Can you work these out from the model? Positions are in its coordinate system, mm. Round coordinates to 2 decimals unless told otherwise and drop trailing zeros. Order: outer loops, then holes, each group sorted by start corner. A loop starts at its lowest first (then second) coordinate and runs counter-clockwise, first axis right, second up.
Q1. If we section it at C-C (y = 7.5): Please give me the cut outline in (x, z), plus the area to 3 significant figures.
Q2. If we section it at A-A (z = 0): Please give me the cut outline in (x, y).
Q3. If we section it at B-B (y = 3.25): Please give me the cut outline in (x, z), plus the area to 3 significant figures.
Q4. If I drill on line 1 (X direction, y = 7.5, z = 0); line 2 (Z direction, x = 1, y = 1.25); line 3 (Z direction, x = 1.5, y = 8), over which ranges is the centre line in solid material (lowest first)?
from build123d import *
from build123d.topology import SkipClean

# Parameters (mm, degrees)
SKETCH1_R                   = 4
BOSS_EXTRUDE1_DEPTH         = 7
F_3_8_24_TAPPED_HOLE6_D     = 8.4328
F_3_8_24_TAPPED_HOLE6_DEPTH = 15.3
F_3_8_24_TAPPED_HOLE6_TIP   = 2.533468714
SKETCH9_R                   = 7.1
SKETCH9_R_2                 = 4.2164
BOSS_EXTRUDE3_DEPTH         = 1.91
FILLET3_R                   = 1
FILLET4_R                   = 0.5


with BuildPart() as part:
    # Sketch1 → Boss-Extrude1 (new body)
    with BuildSketch(Plane(origin=(0, 0, 0), x_dir=(1, 0, 0), z_dir=(0, 1, 0))):
        Polygon((0, 8.198373822), (-7.1, 4.099186911), (-7.1, -4.099186911), (0, -8.198373822), (7.1, -4.099186911), (7.1, 4.099186911), align=None)
        with Locations(Location((0, 0, 0), (0, 0, 270))):
            Circle(SKETCH1_R, mode=Mode.SUBTRACT)
    extrude(amount=BOSS_EXTRUDE1_DEPTH)

    # 3_8-24 Tapped Hole6
    with Locations(Plane.ZX.offset(7)):
        with Locations((0, 0)):
            Hole(F_3_8_24_TAPPED_HOLE6_D / 2, depth=F_3_8_24_TAPPED_HOLE6_DEPTH)
            with Locations((0, 0, -(F_3_8_24_TAPPED_HOLE6_DEPTH + F_3_8_24_TAPPED_HOLE6_TIP / 2))):  # 118° drill point
                Cone(0, F_3_8_24_TAPPED_HOLE6_D / 2, F_3_8_24_TAPPED_HOLE6_TIP, mode=Mode.SUBTRACT)

    # Sketch8 → Cut-Revolve4 (revolve, cut)
    with BuildSketch(Plane.XY, mode=Mode.PRIVATE) as cut_revolve4_sk:
        Polygon((-6.55, -0.5), (-8.05, -0.5), (-11.05, -0.5), (-11.05, 1), (-11.05, 1.5), (-8.55, 1.5), align=None)
        Polygon((-11.05, 5.5), (-11.05, 6), (-11.05, 7.5), (-8.05, 7.5), (-6.55, 7.5), (-8.55, 5.5), align=None)
    revolve(cut_revolve4_sk.sketch.rotate(Axis((0, 0, 0), (0, 1, 0)), 90), axis=Axis((0, 0, 0), (0, 1, 0)), mode=Mode.SUBTRACT)

    # Sketch9 → Boss-Extrude3 (add)
    with SkipClean():  # the faces are left unmerged after this step: merging them gives an invalid solid
        with BuildSketch(Plane(origin=(0, 7, 0), x_dir=(1, 0, 0), z_dir=(0, 1, 0))):
            with Locations(Location((0, 0, 0), (0, 0, 270))):
                Circle(SKETCH9_R)
            with Locations(Location((0, 0, 0), (0, 0, 270))):
                Circle(SKETCH9_R_2, mode=Mode.SUBTRACT)
        extrude(amount=BOSS_EXTRUDE3_DEPTH)
    add(part.part.scale(1), mode=Mode.REPLACE)  # the faces are merged on a copy

    # Fillet3
    fillet3_edges = [part.edges().sort_by_distance(p)[0] for p in [
        (0, 8.91, -7.1),
    ]]
    fillet(fillet3_edges, radius=FILLET3_R)

    # Fillet4
    fillet4_edges = [part.edges().sort_by_distance(p)[0] for p in [
        (0, 8.91, -4.2164),
    ]]
    fillet(fillet4_edges, radius=FILLET4_R)


solid = part.part
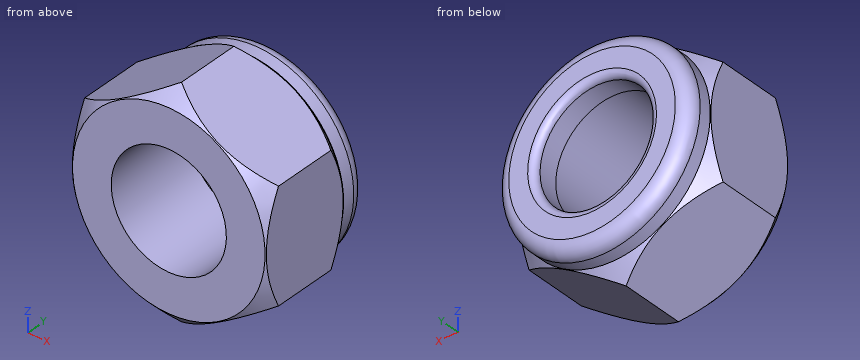
Solution:
1. outline: circle Ø14.2 at (0, 0); hole circle Ø8.43 at (0, 0)
1. area: 103 mm2
2. outline: (-7.1, 0.05) - (-7.05, 0) - (-4.22, 0) - (-4.22, 8.41) arc R0.5 ccw to (-4.72, 8.91) - (-6.1, 8.91) arc R1 ccw to (-7.1, 7.91) - (-7.1, 7) - (-7.05, 7) - (-7.1, 6.95) - close; (4.22, 0) - (7.05, 0) - (7.1, 0.05) - (7.1, 6.95) - (7.05, 7) - (7.1, 7) - (7.1, 7.91) arc R1 ccw to (6.1, 8.91) - (4.72, 8.91) arc R0.5 ccw to (4.22, 8.41) - close
3. outline: (-7.1, -4.1) - (0, -8.2) - (7.1, -4.1) - (7.1, 4.1) - (0, 8.2) - (-7.1, 4.1) - close; hole circle Ø8.43 at (0, 0)
3. area: 119 mm2
4. line 1: x = -7.1 to -4.22, 4.22 to 7.1
4. line 2: z = -7.62 to -4.1, 4.1 to 7.62
4. line 3: z = -6.94 to -3.94, 3.94 to 6.94
